The figure shows three views and two pictorial views of one solid part (mm, origin at its lowest corner). Answer the questions. A direction names the side the tool comes from. Coordinates: 2 decimals unless noted, no trailing zeros. Loops run counter-clockwise (first coordinate to the right, second up) from the corner with the lowest first, then second, coordinate; pieces in that order, holes last. Notation, with made-up numbers: (7, 38) - (11, 38) arc R27 ccw to (11, 59) - close; hole circle Ø9 at (82.5, 48). An arc over 180 degrees is marked (long way). Return JSON: item names as keys, results as strings. Group by question number.
1. Section A-A (z = 5.5) is taken. Write down the section's boundary in (x, y) (1 decimal), and give its area (3 significant figures).
2. Which of the six approach directions +Z, -Z, +X, -X, +Y, -Y give full straight-line access (tool end or side, diameter ignored) to the marked faces 1, 2 and 3?
3. Section C-C (z = 3.25) is taken. Write down the section's boundary in (x, y) (1 decimal).
4. Section B-B (x = 5.3) is taken. Write down the section's boundary in (y, z) (1 decimal).
5. Section D-D (z = 1.25) is taken. Write down the section's boundary in (x, y) (1 decimal).
6. Each of these flat-tipped pins is pushed along its axis until it touches: P1, Ø2.5, axis at y = 3.5, z = 9.5, coming from the +X side; P2, Ø2, axis at y = 2, z = 5, coming from the +X side. Where does it stop, or does it pass through?
7. Find the intervals of material crossed by line 1 along X through (y, z) = (3, 6.75); line 2 along Z through (x, y) = (4.55, 4.9) (1 decimal); line 3 along Z through (x, y) = (3.35, 4.85) (1 decimal), in increasing order.
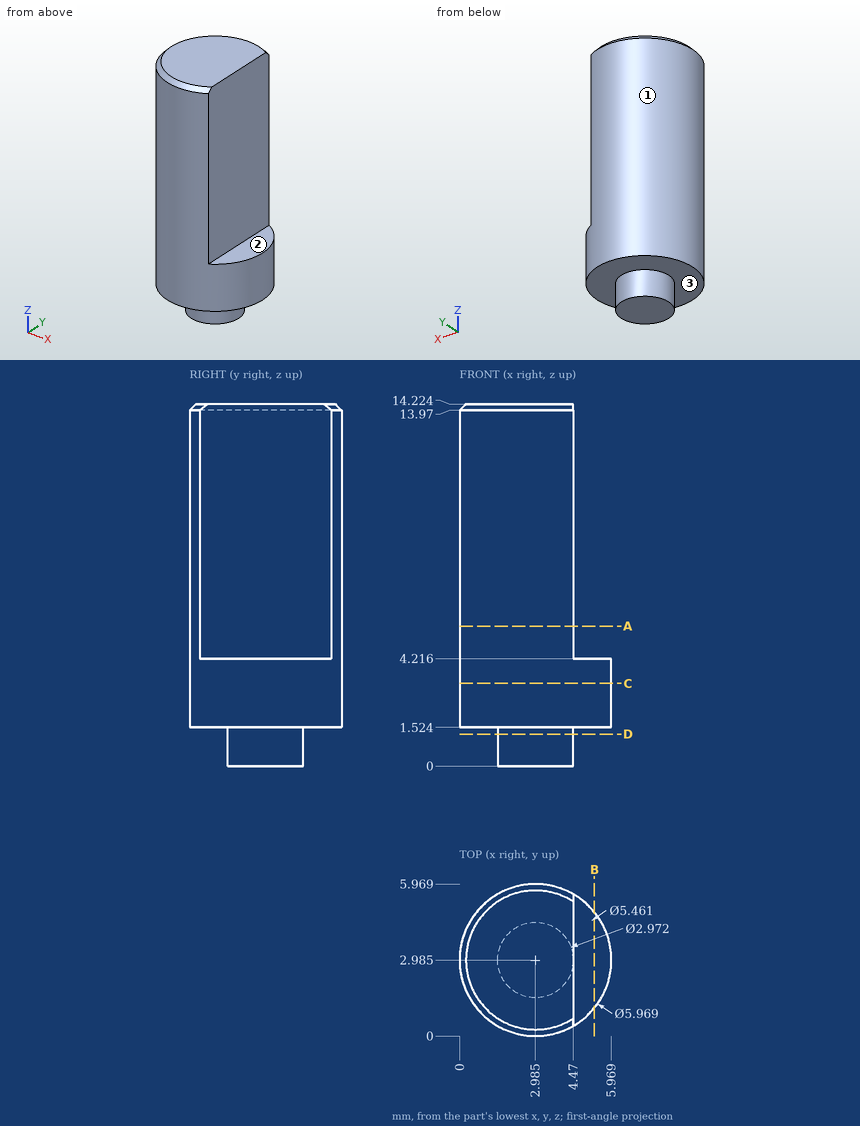
The answers:
{
 "1": {"outline": "(4.5, 0.4) - (4.5, 5.6) arc R3 ccw (long way) to start", "area": "22.5 mm2"},
 "2": {"face 1": "+Z, -Z", "face 2": "+Z, +X, +Y, -Y", "face 3": "-Z"},
 "3": {"outline": "circle Ø6 at (3, 3)"},
 "4": {"outline": "(1.1, 1.5) - (4.9, 1.5) - (4.9, 4.2) - (1.1, 4.2) - close"},
 "5": {"outline": "circle Ø3 at (3, 3)"},
 "6": {"P1": "stops at x = 4.47", "P2": "stops at x = 5.95"},
 "7": {"line 1": "x = 0 to 4.47", "line 2": "z = 1.5 to 4.2", "line 3": "z = 1.5 to 14.2"}
}
